Source: CAD feature listing. Evaluate the final solid. Frame: model axes, mm. Face numbers are marked on the shaded views. A direction names the side the tool comes from. Coordinates: 2 decimals unless noted, no trailing zeros. Write each loop counter-clockwise with the first axis right and the second up, starting at its lowest first coordinate (ties: lowest second). Pieces come first, ordered by that corner, then holes. Notation, with made-up numbers: M -4.5,-8 L 52.5,-8 A26 ccw 52.5,23 Z; hole C 34,88 d11. An arc over 180 degrees is marked long. One line per item, written item: value. Start each with the question number.
Item 1: Cut plane D-D, the plane z = 95. Output: boundary loops of the cut face in (x, y), then the cut area to 3 significant figures.
Item 2: Ray query, L1, parallel to X at y = -87, z = 107; L2, parallel to Z at x = 6, y = -40; L3, parallel to Z at x = 30.5, y = -37. Return the intervals inside material, ascending. Write a range as from..to.
Item 3: Cut plane B-B, the plane z = 16.5. Output: boundary loops of the cut face in (x, y).
Item 4: Cut plane A-A, the plane x = -21. Output: boundary loops of the cut face in (y, z).
Item 5: Set-up query: the marked faces 1, 2 and 3. Return all of +Z, -Z, +X, -X, +Y, -Y with unobstructed straight access to the full face (end or side cutting, diameter ignored); none if empty.
Item 6: Cut plane C-C, the plane y = -3. Output: boundary loops of the cut face in (x, z).
Item 7: Pin query (flat end, axial travel): P1, Ø6, axis at y = -111.5, z = 171.5, coming from the -X side; P2, Ø6.5, axis at y = 5.5, z = 148.5, coming from the +X side; P3, Ø8, axis at x = 19.5, z = 135, coming from the +Y side. Return the tip coordinate at first contact, or that it passes through.
```python
from build123d import *

# Parameters (mm, degrees)
SKETCH_1_W           = 132.33692867
SKETCH_1_H           = 97.034055892
EXTRUDE_1_DEPTH      = 180
SKETCH_2_W           = 37.625025254
SKETCH_2_H           = 34.08860124
SKETCH_2_W_2         = 26.240865703
SKETCH_2_H_2         = 23.4168688
CUT_EXTRUDE_2_DEPTH  = 215.927601009
SKETCH_6_W           = 26.240865703
SKETCH_6_H           = 22.681143593
EXTRUDE_2_DEPTH      = 20
EXTRUDE_3_DEPTH      = 25
EXTRUDE_3_DEPTH_BACK = 25


with BuildPart() as part:
    # Эскиз1 → Бобышка-Вытянуть1 (new body)
    with BuildSketch(Plane.XY):
        with Locations((0, -48.517027946)):
            Rectangle(SKETCH_1_W, SKETCH_1_H)
    extrude(amount=EXTRUDE_1_DEPTH)

    # Эскиз2 → Вырез-Вытянуть2 (cut, through all)
    with BuildSketch(Plane(origin=(0, 0, 0), x_dir=(1, 0, 0), z_dir=(0, 1, 0))):
        with Locations((-18.812512627, -93.188142562)):
            Rectangle(SKETCH_2_W, SKETCH_2_H)
        with Locations((18.812512627, -93.188142562)):
            Rectangle(SKETCH_2_W, SKETCH_2_H)
        with Locations((13.120432852, -11.7084344)):
            Rectangle(SKETCH_2_W_2, SKETCH_2_H_2)
        with Locations((-13.120432852, -11.7084344)):
            Rectangle(SKETCH_2_W_2, SKETCH_2_H_2)
    extrude(amount=-CUT_EXTRUDE_2_DEPTH, mode=Mode.SUBTRACT)

    # Эскиз6 → Бобышка-Вытянуть2 (add)
    with BuildSketch(Plane(origin=(0, -97.034055892, 0), x_dir=(-1, 0, 0), z_dir=(0, -1, 0))):
        with Locations((13.120432852, -168.659428203)):
            Rectangle(SKETCH_6_W, SKETCH_6_H)
        with Locations((-13.120432852, -168.659428203)):
            Rectangle(SKETCH_6_W, SKETCH_6_H)
    extrude(amount=EXTRUDE_2_DEPTH)

    # Эскиз8 → Бобышка-Вытянуть3 (add, two sides: drawn at the far end of the back side and taken through both)
    with BuildSketch(Plane(origin=(0, 0, 0), x_dir=(0, 0, -1), z_dir=(1, 0, 0)).offset(-EXTRUDE_3_DEPTH_BACK)):
        Polygon((-180, 0), (-180, 21.442823519), (-110.232443182, 0), align=None)
    extrude(amount=EXTRUDE_3_DEPTH + EXTRUDE_3_DEPTH_BACK)


solid = part.part
```
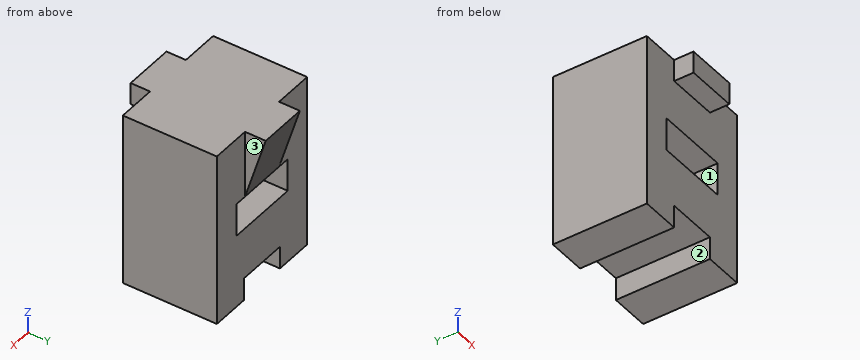
From the geometry:
1. outline: M -66.17,-97.03 L -37.63,-97.03 L -37.63,0 L -66.17,0 Z; M 37.63,-97.03 L 66.17,-97.03 L 66.17,0 L 37.63,0 Z
1. area: 5,540 mm²
2. L1: x = -66.17..-37.63, 37.63..66.17
2. L2: z = 23.42..76.14, 110.23..180
2. L3: z = 0..76.14, 110.23..180
3. outline: M -66.17,-97.03 L -26.24,-97.03 L -26.24,0 L -66.17,0 Z; M 26.24,-97.03 L 66.17,-97.03 L 66.17,0 L 26.24,0 Z
4. outline: M -117.03,157.32 L -97.03,157.32 L -97.03,110.23 L 0,110.23 L 21.44,180 L -117.03,180 Z; M -97.03,23.42 L 0,23.42 L 0,76.14 L -97.03,76.14 Z
5. face 1: +Y, -Y
5. face 2: -Z, +Y, -Y
5. face 3: +Z, -Z, +X, +Y
6. outline: M -66.17,0 L -26.24,0 L -26.24,23.42 L 26.24,23.42 L 26.24,0 L 66.17,0 L 66.17,180 L -66.17,180 Z; hole M -37.63,76.14 L 37.63,76.14 L 37.63,110.23 L -37.63,110.23 Z
7. P1: stops at x = -26.24
7. P2: stops at x = 25
7. P3: stops at y = 8.84
